from build123d import *

# Parameters (mm, degrees)
SKETCH3_R                = 6.35
SKETCH3_R_2              = 1.25
BOSS_EXTRUDE4_DEPTH      = 1.5875
BOSS_EXTRUDE7_DEPTH      = 1.5875
BOSS_EXTRUDE7_DEPTH_BACK = 1.5875
SKETCH9_R                = 6.35
CUT_EXTRUDE3_DEPTH       = 4.175
SKETCH11_W               = 82.024989992
SKETCH11_H               = 3.175
BOSS_EXTRUDE8_DEPTH      = 7.62
SKETCH10_R               = 2.2225
CUT_EXTRUDE4_DEPTH       = 4.175


with BuildPart() as part:
    # Sketch3 → Boss-Extrude4 (new body, symmetric)
    with BuildSketch(Plane(origin=(0, 0, 0), x_dir=(1, 0, 0), z_dir=(0, 1, 0))):
        with BuildLine():
            Line((-25.4, 0), (-25.4, -25.4))
            Line((-25.4, -25.4), (0, -25.4))
            Line((0, -25.4), (25.4, -25.4))
            Line((25.4, -25.4), (25.4, 0))
            ThreePointArc((25.4, 0), (0, 25.4), (-25.4, 0))
        make_face()
        with Locations((0, 7)):
            Circle(SKETCH3_R, mode=Mode.SUBTRACT)
        with Locations((7.75, 13.423393759)):
            Circle(SKETCH3_R_2, mode=Mode.SUBTRACT)
        with Locations((-7.75, 13.423393759)):
            Circle(SKETCH3_R_2, mode=Mode.SUBTRACT)
        with Locations((-7.75, -13.423393759)):
            Circle(SKETCH3_R_2, mode=Mode.SUBTRACT)
        with Locations((7.75, -13.423393759)):
            Circle(SKETCH3_R_2, mode=Mode.SUBTRACT)
    extrude(amount=BOSS_EXTRUDE4_DEPTH, both=True)

    # Sketch8 → Boss-Extrude7 (add, two sides)
    with BuildSketch(Plane(origin=(0, 0, 0), x_dir=(1, 0, 0), z_dir=(0, 1, 0))) as boss_extrude7_sk:
        with BuildLine():
            Line((25.4, -25.4), (25.4, 0))
            ThreePointArc((25.4, 0), (12.395970521, 22.169797357), (-13.300780696, 21.639067283))
            ThreePointArc((-13.300780696, 21.639067283), (15.612494996, 29.814593742), (44.525770688, 21.639067283))
            ThreePointArc((44.525770688, 21.639067283), (53.394787349, 12.395970521), (56.624989992, 0))
            Line((56.624989992, 0), (56.624989992, -25.4))
            Line((56.624989992, -25.4), (25.4, -25.4))
        make_face()
    extrude(amount=BOSS_EXTRUDE7_DEPTH)
    extrude(boss_extrude7_sk.sketch, amount=-BOSS_EXTRUDE7_DEPTH_BACK)

    # Sketch9 → Cut-Extrude3 (cut, through all)
    with BuildSketch(Plane(origin=(0, 1.5875, 0), x_dir=(1, 0, 0), z_dir=(0, 1, 0))):
        with Locations((31.224989992, 0)):
            Circle(SKETCH9_R)
    extrude(amount=-CUT_EXTRUDE3_DEPTH, mode=Mode.SUBTRACT)

    # Sketch11 → Boss-Extrude8 (add)
    with BuildSketch(Plane.XY.offset(25.4)):
        with Locations((15.612494996, 0)):
            Rectangle(SKETCH11_W, SKETCH11_H)
    extrude(amount=BOSS_EXTRUDE8_DEPTH)

    # Sketch10 → Cut-Extrude4 (cut, through all)
    with BuildSketch(Plane(origin=(0, -1.5875, 0), x_dir=(-1, 0, 0), z_dir=(0, -1, 0))):
        with Locations((-15.612494996, -25.0825)):
            Circle(SKETCH10_R)
        with Locations((-48.052489992, -25.0825)):
            Circle(SKETCH10_R)
        with Locations((16.8275, -25.0825)):
            Circle(SKETCH10_R)
    extrude(amount=-CUT_EXTRUDE4_DEPTH, mode=Mode.SUBTRACT)


solid = part.part
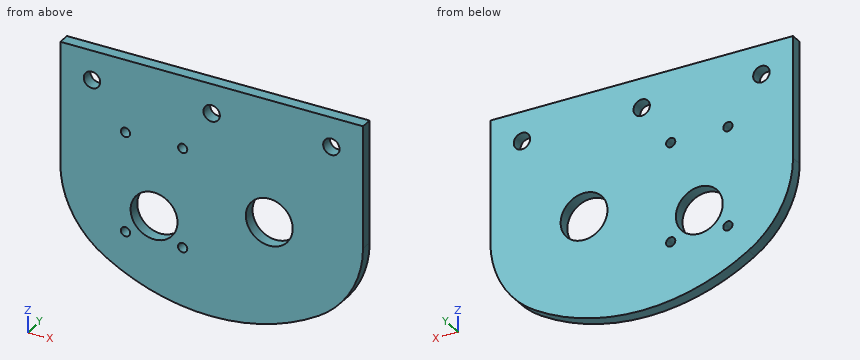
Verification items for the finished model (mm, model axes). Round coordinates to 2 decimals unless told otherwise and drop trailing zeros. Loops run counter-clockwise (first coordinate to the right, second up) from the corner with the lowest first, then second, coordinate; pieces in that order, holes last. Notation, with made-up numbers: (16, 23.25) - (59, 23.25) arc R13 ccw to (59, 31.25) - close; hole circle Ø8 at (56.25, -29.75). An arc over 180 degrees is marked (long way). Write item = value, one per line.
Q1. Sectioned sample at D-D on x = 41. Record the boundary of the cut face in (y, z), plus the area to 3 significant figures.
Here are the results:
outline = (-1.59, -23.63) - (1.59, -23.63) - (1.59, 33.02) - (-1.59, 33.02) - close
area = 180 mm^2
Q2. Sectioned sample at C-C on y = 0.15. State how many separate pieces and enclosed holes the cut face has, plus the area to 3 significant figures.
Here are the results:
separate_pieces = 1
enclosed_holes = 9
area = 4,330 mm^2
Q3. Sectioned sample at B-B on z = -4. Record the boundary of the cut face in (x, y), plus the area to 3 significant figures.
Here are the results:
outline = (-25.08, -1.59) - (-5.6, -1.59) - (-5.6, 1.59) - (-25.08, 1.59) - close; (5.6, -1.59) - (26.29, -1.59) - (26.29, 1.59) - (5.6, 1.59) - close; (36.16, -1.59) - (56.31, -1.59) - (56.31, 1.59) - (36.16, 1.59) - close
area = 192 mm^2
Q4. Material ranges on L1, parallel to X at y = -1, z = 25; L2, parallel to Z at x = 48, y = -0.4; L3, parallel to X at y = -1.4, z = 26.5, recorded low to high.
Here are the results:
L1 = -25.4 to -19.05, -14.61 to 13.39, 17.83 to 45.83, 50.27 to 56.62
L2 = -19.07 to 22.86, 27.3 to 33.02
L3 = -25.4 to -18.54, -15.12 to 13.9, 17.32 to 46.34, 49.76 to 56.62
Q5. Depth check by flat-ended pin: pin 1 (4 mm diameter, centred on x = 7.75, z = -13.42, fed in from -Y); pin 2 (1.5 mm diameter, centred on x = 46, y = 1, fed in from -Z); pin 3 (10 mm diameter, centred on x = 31.22, z = 0, fed in from -Y). Enter the tip coordinate at first touch or a pass-through.
Here are the results:
pin_1 = -1.59
pin_2 = -21.18
pin_3 = through
Q6. Sectioned sample at A-A on x = 0. Record the boundary of the cut face in (y, z).
Here are the results:
outline = (-1.59, -27.56) - (1.59, -27.56) - (1.59, -13.35) - (-1.59, -13.35) - close; (-1.59, -0.65) - (1.59, -0.65) - (1.59, 33.02) - (-1.59, 33.02) - close
